The listing builds one solid part. Answer for the finished solid, in the listing's coordinates (mm). Coordinates: 2 decimals unless noted, no trailing zeros. Loops run counter-clockwise (first coordinate to the right, second up) from the corner with the lowest first, then second, coordinate; pieces in that order, holes last. Notation, with made-up numbers: M -4.5,19.25 L 42.5,19.25 A28 cw 42.5,52.25 Z; hole C -38.5,-9.75 d8. An arc over 180 degrees is marked long. Answer as a JSON object with one key per item and string values. Group by question number.
1. A cutting plane is placed at A-A on y = -55.5. Give the vertices of the cut face in (x, z), and give its area (3 significant figures).
2. Straight lines are drawn through the part: L1, parallel to X at y = -4.5, z = 3.9; L2, parallel to X at y = -44, z = 3.05; L3, parallel to Y at x = -59, z = 1.9. For each, find the intervals that lie inside material, in ascending order.
3. Given pin 1 (1 mm diameter, centred on x = -158, z = 1.5, fed in from -Y), flat-ended and moving along its own axis, determine where the tip first touches the part or whether it passes through.
4. A cutting plane is placed at B-B on z = 2.1. State how many separate pieces and enclosed holes the cut face has, and give its area (3 significant figures).
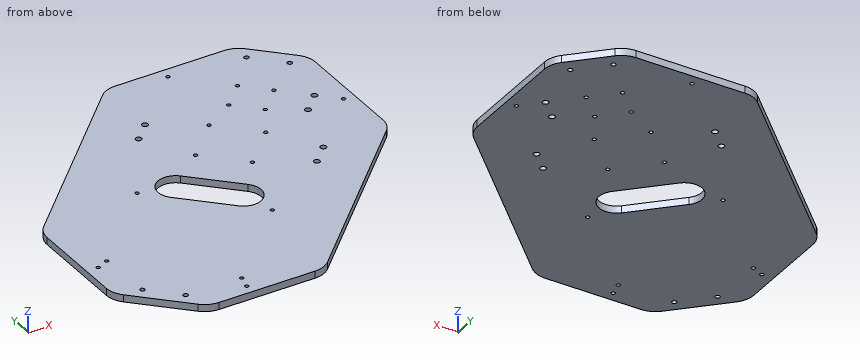
from build123d import *

# Parameters (mm, degrees)
SKETCH1_R           = 2
SKETCH1_R_2         = 1.6
SKETCH1_R_3         = 2.5
BOSS_EXTRUDE1_DEPTH = 6


with BuildPart() as part:
    # Sketch1 → Boss-Extrude1 (new body)
    with BuildSketch(Plane.XY):
        with BuildLine():
            Line((-209.57060205, 21.0430454), (-79.778754851, 150.834892598))
            ThreePointArc((-79.778754851, 150.834892598), (-73.290287875, 155.170347624), (-65.636619228, 156.692756974))
            Line((-65.636619228, 156.692756974), (26.789787643, 156.692756974))
            ThreePointArc((26.789787643, 156.692756974), (34.443456291, 155.170347624), (40.931923267, 150.834892598))
            Line((40.931923267, 150.834892598), (68.713669198, 123.053146667))
            ThreePointArc((68.713669198, 123.053146667), (73.049124224, 116.564679691), (74.571533574, 108.911011044))
            Line((74.571533574, 108.911011044), (74.571533574, 16.484604172))
            ThreePointArc((74.571533574, 16.484604172), (73.049124224, 8.830935525), (68.713669198, 2.342468549))
            Line((68.713669198, 2.342468549), (-61.078178001, -127.44937865))
            ThreePointArc((-61.078178001, -127.44937865), (-67.566644977, -131.784833676), (-75.220313624, -133.307243026))
            Line((-75.220313624, -133.307243026), (-156.333011997, -133.307243026))
            ThreePointArc((-156.333011997, -133.307243026), (-163.986680644, -131.784833676), (-170.47514762, -127.44937865))
            Line((-170.47514762, -127.44937865), (-209.57060205, -88.35392422))
            ThreePointArc((-209.57060205, -88.35392422), (-213.906057076, -81.865457244), (-215.428466426, -74.211788596))
            Line((-215.428466426, -74.211788596), (-215.428466426, 6.900909776))
            ThreePointArc((-215.428466426, 6.900909776), (-213.906057076, 14.554578423), (-209.57060205, 21.0430454))
        make_face()
        with Locations((-194.265515522, -89.516875124)):
            Circle(SKETCH1_R, mode=Mode.SUBTRACT)
        with Locations((-171.638098524, -112.144292122)):
            Circle(SKETCH1_R, mode=Mode.SUBTRACT)
        with Locations((-195.679729085, -42.847827566)):
            Circle(SKETCH1_R_2, mode=Mode.SUBTRACT)
        with Locations((-124.969050966, -113.558505684)):
            Circle(SKETCH1_R_2, mode=Mode.SUBTRACT)
        with Locations((-57.793906753, -46.383361472)):
            Circle(SKETCH1_R_2, mode=Mode.SUBTRACT)
        with Locations((-128.504584872, 24.327316647)):
            Circle(SKETCH1_R_2, mode=Mode.SUBTRACT)
        with Locations((-205.566364073, -47.103328201)):
            Circle(SKETCH1_R_2, mode=Mode.SUBTRACT)
        with Locations((-127.784618142, -124.885074131)):
            Circle(SKETCH1_R_2, mode=Mode.SUBTRACT)
        with Locations((-65.572081346, 46.247626864)):
            Circle(SKETCH1_R_2, mode=Mode.SUBTRACT)
        with Locations((-35.873596536, 16.549142054)):
            Circle(SKETCH1_R_2, mode=Mode.SUBTRACT)
        with Locations((-6.175111727, 46.247626864)):
            Circle(SKETCH1_R_2, mode=Mode.SUBTRACT)
        with Locations((-35.873596536, 75.946111674)):
            Circle(SKETCH1_R_2, mode=Mode.SUBTRACT)
        with Locations((-9.357092242, 91.85601425)):
            Circle(SKETCH1_R_2, mode=Mode.SUBTRACT)
        with Locations((9.73479085, 72.764131158)):
            Circle(SKETCH1_R_2, mode=Mode.SUBTRACT)
        with Locations((28.826673942, 91.85601425)):
            Circle(SKETCH1_R_2, mode=Mode.SUBTRACT)
        with Locations((9.73479085, 110.947897342)):
            Circle(SKETCH1_R_2, mode=Mode.SUBTRACT)
        with Locations((35.547065377, 140.295705776)):
            Circle(SKETCH1_R, mode=Mode.SUBTRACT)
        with Locations((58.174482375, 117.668288778)):
            Circle(SKETCH1_R, mode=Mode.SUBTRACT)
        with Locations((50.039877378, 70.642810815)):
            Circle(SKETCH1_R_3, mode=Mode.SUBTRACT)
        with Locations((35.897741754, 56.500675191)):
            Circle(SKETCH1_R_3, mode=Mode.SUBTRACT)
        with Locations((18.573625615, 7.356753899)):
            Circle(SKETCH1_R_3, mode=Mode.SUBTRACT)
        with Locations((4.431489991, -6.785381725)):
            Circle(SKETCH1_R_3, mode=Mode.SUBTRACT)
        with Locations((-74.764469502, 100.694849015)):
            Circle(SKETCH1_R_3, mode=Mode.SUBTRACT)
        with Locations((-88.906605125, 86.552713392)):
            Circle(SKETCH1_R_3, mode=Mode.SUBTRACT)
        with Locations((-26.494483604, 147.55062135)):
            Circle(SKETCH1_R_2, mode=Mode.SUBTRACT)
        with Locations((65.42939795, 55.626739796)):
            Circle(SKETCH1_R_2, mode=Mode.SUBTRACT)
        with BuildLine():
            Line((-89.613711907, 27.862850553), (-54.258372847, -7.492488506))
            ThreePointArc((-54.258372847, -7.492488506), (-54.258372847, -28.705691942), (-75.471576283, -28.705691942))
            Line((-75.471576283, -28.705691942), (-110.826915342, 6.649647117))
            ThreePointArc((-110.826915342, 6.649647117), (-110.826915342, 27.862850553), (-89.613711907, 27.862850553))
        make_face(mode=Mode.SUBTRACT)
    extrude(amount=BOSS_EXTRUDE1_DEPTH)


solid = part.part
From the geometry:
{
 "1": {"outline": "M -215.43,0 L 10.87,0 L 10.87,6 L -215.43,6 Z", "area": "1,360 mm²"},
 "2": {"L1": "x = -215.43 to -99.68, -57.25 to 3.42, 5.44 to 61.87", "L2": "x = -215.43 to -196.79, -194.57 to 22.37", "L3": "y = -125.37 to -47.43, -45.33 to -31.9, -2.75 to 156.69"},
 "3": {"pin 1": "stops at y = -133.27"},
 "4": {"separate pieces": "1", "enclosed holes": "27", "area": "59,400 mm²"}
}
